from build123d import *

# Parameters (mm, degrees)
SKETCH1_R                = 1.65
BOSS_EXTRUDE1_DEPTH      = 3
BOSS_EXTRUDE2_DEPTH      = 2
BOSS_EXTRUDE2_DEPTH_BACK = 2
SKETCH2_W                = 3.107139826
SKETCH2_H                = 1.36
FILLET1_R                = 0.25


with BuildPart() as part:
    # Sketch1 → Boss-Extrude1 (new body)
    with BuildSketch(Plane(origin=(0, 0, 0), x_dir=(0, 1, 0), z_dir=(0, 0, 1))):
        with BuildLine():
            Line((-3.75, 0), (-3.75, 5.743917642))
            Line((-3.75, 5.743917642), (3.75, 5.743917642))
            Line((3.75, 5.743917642), (3.75, 0))
            ThreePointArc((3.75, 0), (0, -3.75), (-3.75, 0))
        make_face()
        with Locations(Location((0, 0, 0), (0, 0, 270))):
            Circle(SKETCH1_R, mode=Mode.SUBTRACT)
    extrude(amount=BOSS_EXTRUDE1_DEPTH)

    # Sketch2 → Boss-Extrude2 (add, two sides: drawn at the far end of the back side and taken through both)
    with BuildSketch(Plane(origin=(0, 0, 0), x_dir=(-1, 0, 0), z_dir=(0, 1, 0)).offset(-BOSS_EXTRUDE2_DEPTH_BACK)):
        with Locations((7.297487555, 2.32)):
            Rectangle(SKETCH2_W, SKETCH2_H)
    extrude(amount=BOSS_EXTRUDE2_DEPTH + BOSS_EXTRUDE2_DEPTH_BACK)

    # Fillet1
    fillet1_edges = [part.edges().sort_by_distance(p)[0] for p in [
        (-1.65, 0, 0),
        (-1.65, 0, 3),
        (-5.743917642, 2.875, 3),
        (-2.871958821, -3.75, 3),
        (-5.743917642, -2.875, 3),
        (-5.743917642, -2, 2.32),
        (-5.743917642, 0, 1.64),
        (-7.297487555, -2, 1.64),
        (-8.851057468, 0, 1.64),
        (-8.851057468, -2, 2.32),
        (-8.851057468, 0, 3),
        (-7.297487555, -2, 3),
        (-5.743917642, 2, 2.32),
        (-7.297487555, 2, 1.64),
        (-8.851057468, 2, 2.32),
        (-7.297487555, 2, 3),
        (3.75, 0, 3),
        (-2.871958821, -3.75, 0),
        (-5.743917642, 0, 0),
        (-2.871958821, 3.75, 0),
        (3.75, 0, 0),
        (-5.743917642, -3.75, 1.5),
        (-5.743917642, 3.75, 1.5),
        (-2.871958821, 3.75, 3),
    ]]
    fillet(fillet1_edges, radius=FILLET1_R)


solid = part.part
Check sheet for the modelled part. Datum: model origin and axes. Units: mm. A direction names the side the tool comes from. Round coordinates to 2 decimals unless told otherwise and drop trailing zeros. Loops run counter-clockwise (first coordinate to the right, second up) from the corner with the lowest first, then second, coordinate; pieces in that order, holes last. Notation, with made-up numbers: M 85.5,-7.5 L 120.5,-7.5 A30 ccw 120.5,27.5 Z; hole C 73.5,10.5 d9. An arc over 180 degrees is marked long. One line per item, written item: value.
(1) Release check for a two-part mould opening along X. For faces 5 (the face through (-1.31, -1, 1.48)), 6 (the face through (-5.744, 0, 1)), 7 (the face through (-3, 0, 3)) record: +X half, -X half, draft (parallel to the pull), parting line (faces both ways), or undercut.
Computed values:
face 5: undercut
face 6: -X half
face 7: draft
(2) Access from +Z, -Z, +X, -X, +Y, -Y to the whole of each face (thin tool, end or side, straight path). Record for faces 1 (the face through (-8.851, 0, 2.3)), 2 (the face through (-7.3, -2, 2.3)), 3 (the face through (-7, 0, 1.64)), 4 (the face through (-7.3, 2, 2.3)).
Computed values:
face 1: +Z, -Z, -X, +Y, -Y
face 2: +Z, -Z, -X, -Y
face 3: -Z, -X, +Y, -Y
face 4: +Z, -Z, -X, +Y
(3) Depth check by flat-ended pin: pin 1 Ø1.3 at (x, y) = (-7, -0.5) entering from -Z; pin 2 Ø1.5 at (y, z) = (-3, 1) entering from +X. Enter the tip coordinate at first touch or a pass-through.
Computed values:
pin 1: stops at z = 1.64
pin 2: stops at x = 3
(4) Sectioned sample at A-A, the plane y = 0. Record the cut outline in (x, z), then the cut area to 3 significant figures.
Computed values:
outline: M -8.85,1.89 A0.25 ccw -8.6,1.64 L -5.99,1.64 A0.25 cw -5.74,1.39 L -5.74,0.25 A0.25 ccw -5.49,0 L -1.9,0 A0.25 ccw -1.65,0.25 L -1.65,2.75 A0.25 ccw -1.9,3 L -8.6,3 A0.25 ccw -8.85,2.75 Z; M 1.65,0.25 A0.25 ccw 1.9,0 L 3.5,0 A0.25 ccw 3.75,0.25 L 3.75,2.75 A0.25 ccw 3.5,3 L 1.9,3 A0.25 ccw 1.65,2.75 Z
area: 22.7 mm^2
(5) Thickness scan on line 1 (X direction, y = -2.25, z = 0.4); line 2 (X direction, y = 0.5, z = 2.1); line 3 (X direction, y = -1.25, z = 2.7). Record the ranges inside material, lowest first.
Computed values:
line 1: x = -5.74 to 3
line 2: x = -8.85 to -1.57, 1.57 to 3.72
line 3: x = -8.85 to -1.08, 1.08 to 3.54
